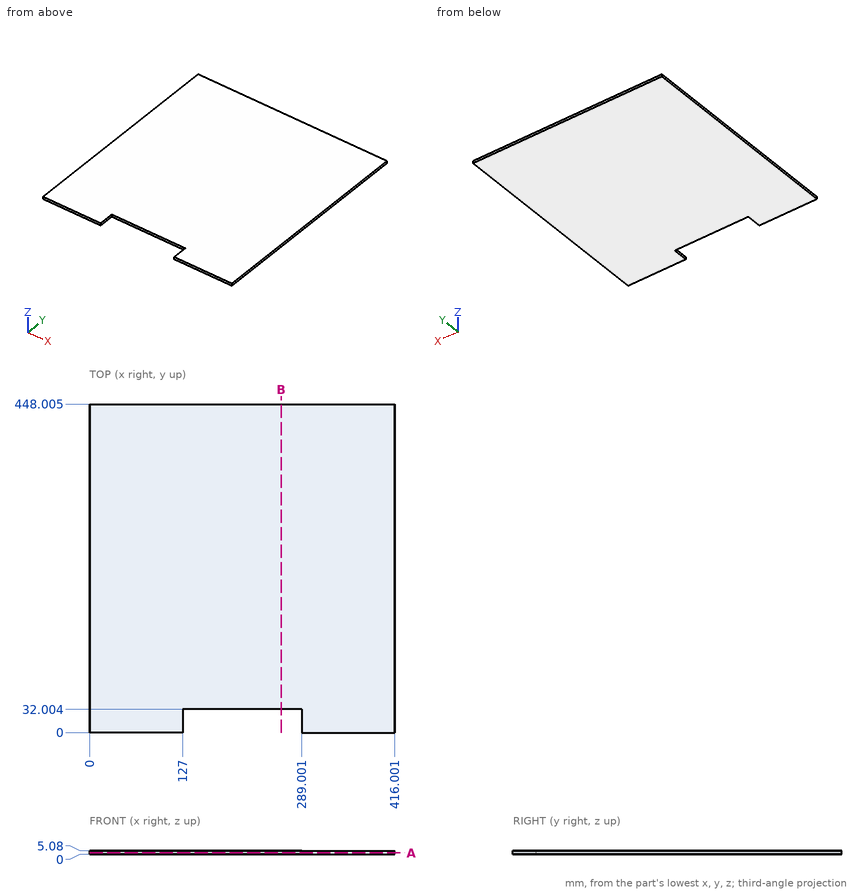
Job drawing, mm, ordinate dimensions from the low corner. One solid piece. Give positions to 0.01 mm unless a question says otherwise; leave off trailing zeros. Loops run counter-clockwise (first coordinate to the right, second up) from the corner with the lowest first, then second, coordinate; pieces in that order, holes last. Notation, with made-up numbers: M 84.5,11.5 L 119.5,11.5 A20 ccw 119.5,49.5 Z; hole C 61,-9 d5. An arc over 180 degrees is marked long. Return JSON: item names as keys, results as strings.
1) Drill centre line: line 1 (Y direction, x = 263, z = 4.45) (1 decimal). Where is it in solid material? Low to high.
Calculated:
{"line 1": "y = 32 to 448"}
2) Saw through at A-A, the plane z = 2.25. List the corners of the cut face in (x, y) (1 decimal), then the cut area to 3 significant figures.
Calculated:
{"outline": "M 0,0 L 127,0 L 127,32 L 289,32 L 289,0 L 416,0 L 416,448 L 0,448 Z", "area": "181,000 mm2"}
3) Saw through at B-B, the plane x = 261. List the corners of the cut face in (y, z) (1 decimal).
Calculated:
{"outline": "M 32,0 L 448,0 L 448,5.1 L 32,5.1 Z"}
4) Flat gauge pin, fed straight in: pin 1 Ø2 at (x, z) = (247.5, 1) entering from -Y. Where does the tip first touch, or does it go through?
Calculated:
{"pin 1": "stops at y = 32"}
